```python
from build123d import *

# Parameters (mm, degrees)
F3_DEPTH = 25.4
F4_T     = -2.54


# Not quite as in the source:
# - the program builds the solid bodies; features that only make, move or delete a surface that nothing else refers to are left out


with BuildPart() as f3:
    # F2 (on Front) → F3 (new body)
    with BuildSketch(Plane.XZ):
        Polygon((3.7617208479, 48.2991386944), (-44.7727749167, 18.5028637951), (-31.4328175171, -36.8637399798), (25.346225329, -41.2859080551), (47.0976462569, 11.3476455454), align=None)
    extrude(amount=F3_DEPTH)

    # F4
    f4_openings = [f3.faces().sort_by_distance(p)[0] for p in [
        (0, 0, 0),
    ]]
    offset(amount=F4_T, openings=f4_openings)


solid = f3.part
```
Verification items for the finished model (mm, model axes). A direction names the side the tool comes from. Coordinates: 2 decimals unless noted, no trailing zeros. Order: outer loops, then holes, each group sorted by start corner. A loop starts at its lowest first (then second) coordinate and runs counter-clockwise, first axis right, second up. Notation, with made-up numbers: (70, 62.5) -> (120, 62.5) arc R26 cw to (120, 89.5) -> close; hole circle Ø11 at (83, 47.5). An arc over 180 degrees is marked (long way). Answer as CSV lines item,"result". Start each with the question number.
1) Release check for a two-part mould opening along X. For faces 3 (the face through (35, 0, -13)), 4 (the face through (-20.166, -12.522, 33.61)), 5 (the face through (25.733, -12.522, 29.565)), 6 (the face through (33.732, -11.27, -14.344)) record: released by +X, released by -X, zero draft, split by the parting line, or undercut.
2) Set-up check for faces 1 (the face through (-38.196, -12.522, -8.793)), 2 (the face through (-18.86, -11.27, 31.43)): record each of +Z, -Z, +X, -X, +Y, -Y from which the full face is reachable in a straight line by a thin tool's end or side.
3) Cross-section at B-B, the plane z = 29. Record the boundary of the cut face in (x, y).
4) Material ranges on L1, parallel to Y at x = 23, z = 20.5; L2, parallel to X at y = -21.5, z = 20; L3, parallel to X at y = -0.75, z = 44, recorded low to high. Write a range as [from, to].
5) Gauge pin test, flat ends, axial feed: pin 1 Ø5 at (x, y) = (-29, -10.5) entering from -Z; pin 2 Ø1 at (x, z) = (-4.5, 4) entering from +Y; pin 3 Ø12 at (y, z) = (-10.5, 11.5) entering from -X. Record the tip position at first contact, or that the pin passes through.
6) Cross-section at A-A, the plane y = -20.5. Record the boundary of the cut face in (x, z).
7) Cross-section at C-C, the plane x = -22. Record the boundary of the cut face in (y, z).
Conclusion:
1,face 3,"zero draft"
1,face 4,"released by -X"
1,face 5,"released by +X"
1,face 6,"undercut"
2,face 1,"-Z, -X, +Y, -Y"
2,face 2,"+Y"
3,outline,"(-27.67, -25.4) -> (26.4, -25.4) -> (26.4, 0) -> (22.48, 0) -> (22.48, -22.86) -> (-22.82, -22.86) -> (-22.82, 0) -> (-27.67, 0) -> close"
4,L1,"y = [-25.4, -22.86]"
4,L2,"x = [-42.33, -37.48], [33.04, 36.95]"
4,L3,"x = [-3.24, 1.61], [4.89, 8.8]"
5,pin 1,"stops at z = -37.25"
5,pin 2,"stops at y = -22.86"
5,pin 3,"stops at x = -44.53"
6,outline,"(-44.77, 18.5) -> (-31.43, -36.86) -> (25.35, -41.29) -> (47.1, 11.35) -> (3.76, 48.3) -> close; hole (-41.87, 17.3) -> (-29.4, -34.47) -> (23.7, -38.61) -> (44.05, 10.61) -> (3.52, 45.17) -> close"
7,outline,"(-25.4, -37.6) -> (0, -37.6) -> (0, -35.05) -> (-22.86, -35.05) -> (-22.86, 29.5) -> (0, 29.5) -> (0, 32.48) -> (-25.4, 32.48) -> close"
